Model file for the job. Use its own axes, mm. Round coordinates to 2 decimals unless told otherwise and drop trailing zeros. Loops run counter-clockwise (first coordinate to the right, second up) from the corner with the lowest first, then second, coordinate; pieces in that order, holes last. Notation, with made-up numbers: M 76,76.25 L 123,76.25 A9 cw 123,82.25 Z; hole C 21.5,32 d5. An arc over 180 degrees is marked long. Use a Markdown table: item, result. Add a question column.
Q1. Cut at C-C (z = 5). Give the cut face in (x, y).
Q2. Cut at D-D (z = 26). Give the cut face in (x, y), plus the area to 3 significant figures.
Q3. Cut at A-A (y = 0). Give the cut face in (x, z).
Q4. Pin check, flat tips, straight feed: pin 1 (3 mm diameter, centred on y = -2, z = 30, fed in from -X); pin 2 (5 mm diameter, centred on x = -3.5, z = 35, fed in from -Y); pin 3 (6 mm diameter, centred on x = 6, z = 12.5, fed in from +Y). Stop position of each tip, or through.
Q5. Probe line 1 (Z direction, x = 2.75, y = -6); line 2 (Z direction, x = 4, y = -4); line 3 (Y direction, x = 4.75, z = 39.5). List the from-to ranges inside material, lowest first. Write a range as from..to.
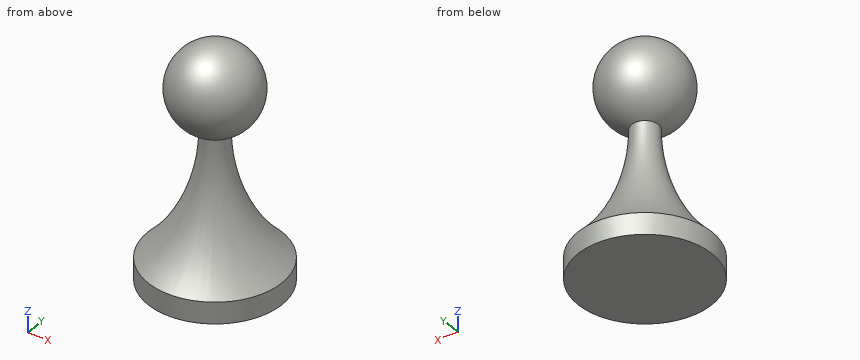
from build123d import *


# Not quite as in the source:
# - a feature of the source that left no trace in its solid (it failed there, or was rolled back) is left out


with BuildPart() as f1:
    # F0 (on Front) → F1 (revolve)
    with BuildSketch(Plane.XZ):
        with BuildLine():
            ThreePointArc((-2.5, 27.4883110198), (-1.2659509046, 27.1884526113), (0, 27.0876530966))
            Line((0, 27.0876530966), (0, 43.0876530966))
            ThreePointArc((0, 43.0876530966), (-7.8992004853, 36.3536040012), (-2.5, 27.4883110198))
        make_face()
    revolve(axis=Axis((0, 0, 35.0876530966), (0, 0, -1)))

    # F0 (on Front) → F2 (revolve)
    with BuildSketch(Plane.XZ):
        with BuildLine():
            ThreePointArc((-2.5, 27.4883110198), (-5.1040521689, 14.7240958602), (-12.5, 4))
            Line((-12.5, 4), (-2.5, 4))
            Line((-2.5, 4), (-2.5, 27.4883110198))
        make_face()
        with BuildLine():
            Line((-2.5, 4), (0, 4))
            Line((0, 4), (0, 27.0876530966))
            ThreePointArc((0, 27.0876530966), (-1.2659509046, 27.1884526113), (-2.5, 27.4883110198))
            Line((-2.5, 27.4883110198), (-2.5, 4))
        make_face()
    revolve(axis=Axis((0, 0, 15.5438265483), (0, 0, -1)))

    # F0 (on Front) → F3 (revolve)
    with BuildSketch(Plane.XZ):
        Polygon((-12.5, 0), (0, 0), (0, 4), (-2.5, 4), (-12.5, 4), align=None)
        with BuildLine():
            Line((-2.5, 4), (0, 4))
            Line((0, 4), (0, 27.0876530966))
            ThreePointArc((0, 27.0876530966), (-1.2659509046, 27.1884526113), (-2.5, 27.4883110198))
            Line((-2.5, 27.4883110198), (-2.5, 4))
        make_face()
    revolve(axis=Axis((0, 0, 2), (0, 0, 1)))


solid = f1.part
Checked values:
| question | item | result |
|---|---|---|
| 1 | outline | C 0,0 d23.01 |
| 2 | outline | C 0,0 d5.07 |
| 2 | area | 20.2 mm^2 |
| 3 | outline | M -12.5,0 L 12.5,0 L 12.5,4 A32.59 cw 2.5,27.49 A8 ccw long -2.5,27.49 A32.59 cw -12.5,4 Z |
| 4 | pin 1 | stops at x = -6.95 |
| 4 | pin 2 | stops at y = -7.94 |
| 4 | pin 3 | stops at y = 6.26 |
| 5 | line 1 | z = 0..11.66, 30.57..39.61 |
| 5 | line 2 | z = 0..13.5, 29.43..40.74 |
| 5 | line 3 | y = -4.69..4.69 |
